```python
from build123d import *

# Parameters (mm, degrees)
BOSS_EXTRUDE1_DEPTH = 3.175
SKETCH2_W           = 25.4
SKETCH2_H           = 2.38125
BOSS_EXTRUDE2_DEPTH = 3.175
CUT_EXTRUDE1_DEPTH  = 4.175
FILLET1_R           = 9.525
FILLET2_R           = 63.5


with BuildPart() as part:
    # Sketch1 → Boss-Extrude1 (new body)
    with BuildSketch(Plane(origin=(0, 0, 0), x_dir=(1, 0, 0), z_dir=(0, 1, 0))):
        Polygon((-50.8, 0), (0, 0), (46.040435581, 21.469007696), (40.673183657, 32.979116592), (-50.8, 12.7), align=None)
    extrude(amount=BOSS_EXTRUDE1_DEPTH)

    # Sketch2 → Boss-Extrude2 (add)
    with BuildSketch(Plane(origin=(0, 3.175, 0), x_dir=(1, 0, 0), z_dir=(0, 1, 0))):
        Polygon((23.020217791, 10.734503848), (46.040435581, 21.469007696), (47.046795317, 19.310862279), (24.026577527, 8.57635843), align=None)
        with Locations((-38.1, -1.190625)):
            Rectangle(SKETCH2_W, SKETCH2_H)
    extrude(amount=-BOSS_EXTRUDE2_DEPTH)

    # Sketch3 → Cut-Extrude1 (cut, through all)
    with BuildSketch(Plane(origin=(0, 3.175, 0), x_dir=(1, 0, 0), z_dir=(0, 1, 0))):
        Polygon((-25.4, 11.43), (-50.8, 11.43), (-50.8, 12.7), (40.673183657, 32.979116592), (41.20990885, 31.828105702), (18.189691059, 21.093601854), (-2.533969994, 11.43), align=None)
    extrude(amount=-CUT_EXTRUDE1_DEPTH, mode=Mode.SUBTRACT)

    # Fillet1
    fillet1_edges = [part.edges().sort_by_distance(p)[0] for p in [
        (0, 1.5875, 0),
        (41.20990885, 1.5875, -31.828105702),
        (-50.8, 1.5875, -11.43),
    ]]
    fillet(fillet1_edges, radius=FILLET1_R)

    # Fillet2
    fillet2_edges = [part.edges().sort_by_distance(p)[0] for p in [
        (-2.533969994, 1.5875, -11.43),
    ]]
    fillet(fillet2_edges, radius=FILLET2_R)


solid = part.part
```
Geometry: final body of the model. Coordinates: model frame, mm. A direction names the side the tool comes from. Round coordinates to 2 decimals unless told otherwise and drop trailing zeros. Order: outer loops, then holes, each group sorted by start corner. A loop starts at its lowest first (then second) coordinate and runs counter-clockwise, first axis right, second up. Notation, with made-up numbers: (7.5, 71.5) - (25.5, 71.5) arc R21 ccw to (25.5, 96.5) - close; hole circle Ø8 at (-22, 72). An arc over 180 degrees is marked (long way). Use CSV: the item, a comma, the result in double quotes. Start each with the question number.
Q1. Material intervals for line 1 along Z through (x, y) = (-38, 2.65); line 2 along Z through (x, y) = (-21, 0.6); line 3 along X through (y, z) = (2.55, -5.5), sorted ascending. Write a range as from..to.
Q2. Access query for faces 1 (the face through (-38, 2, 2.381)), 2 (the face through (12.319, 1.565, -5.745)), 3 (the face through (-1, 3.175, -10)), 4 (the face through (-25.4, 2, 1)), 5 (the face through (-29, 2, -11.43)). Directions: +Z, -Z, +X, -X, +Y, -Y. A direction counts if a zero-diameter tool reaches every point of the face in a straight line with its end or side. Return the directions, or none.
Q3. Mould query, pull axis X, two halves, no side actions, for faces 6 (the face through (23.53, 1.61, -9.64)), 7 (the face through (-2.678, 1.565, -12.977)), 8 (the face through (35.7, 1.61, -14.02)). Classes: +X half, -X half, draft (parallel to the pull), parting line (faces both ways), or undercut.
Q4. First-contact query: pin 1 (1.5 mm diameter, centred on x = 22, y = 1, fed in from +Z); pin 2 (0.7 mm diameter, centred on y = 1.5, z = 1.5, fed in from +X); pin 3 (1 mm diameter, centred on x = -14, y = 1, fed in from +Z). Flat tips, straight axial feed; report the tip coordinate or a pass-through.
Q5. Section query C-C (z = -4.5). Return loops of the section in (x, y) (3 decimals), and give its area (3 significant figures).
Q6. Section query B-B (x = -19). Return loops of the section in (y, z) (3 decimals), and give its area (3 significant figures).
Result set:
1,line 1,"z = -11.43..2.38"
1,line 2,"z = -11.43..0"
1,line 3,"x = -50.1..11.79"
2,face 1,"+Z, +X, -X, +Y, -Y"
2,face 2,"+Z, +Y, -Y"
2,face 3,"+Z, -Z, +X, -X, +Y"
2,face 4,"+Z, +X, +Y, -Y"
2,face 5,"-Z, -X, +Y, -Y"
3,face 6,"undercut"
3,face 7,"-X half"
3,face 8,"+X half"
4,pin 1,"stops at z = -9.91"
4,pin 2,"stops at x = -25.4"
4,pin 3,"stops at z = 0"
5,outline,"(-50.44, 0) - (9.65, 0) - (9.65, 3.175) - (-50.44, 3.175) - close"
5,area,"191 mm2"
6,outline,"(0, -11.43) - (3.175, -11.43) - (3.175, 0) - (0, 0) - close"
6,area,"36.3 mm2"
